from build123d import *

# Parameters (mm, degrees)
F0_R     = 25.4
F0_R_2   = 3.81
F1_DEPTH = 6.35
F2_R     = 19.05
F2_R_2   = 13.97
F3_DEPTH = 2.54
F4_R     = 2.53999


# Not quite as in the source:
# - a fillet or chamfer is up to 0.001 mm smaller than in the source, because OpenCascade refuses the exact size


with BuildPart() as f1:
    # F0 (on Front) → F1 (new body)
    with BuildSketch(Plane.XZ):
        Circle(F0_R)
        Circle(F0_R_2, mode=Mode.SUBTRACT)
    extrude(amount=F1_DEPTH)

    # F2 (on face) → F3 (cut)
    with BuildSketch(Plane.XZ.offset(6.35)):
        Circle(F2_R)
        Circle(F2_R_2, mode=Mode.SUBTRACT)
    extrude(amount=-F3_DEPTH, mode=Mode.SUBTRACT)

    # F4 (radius 2.54 in the source; OpenCascade refuses exactly that, so slightly less here)
    f4_edges = [f1.edges().sort_by_distance(p)[0] for p in [
        (-19.05, -3.81, 0),
        (-13.97, -3.81, 0),
    ]]
    fillet(f4_edges, radius=F4_R)


solid = f1.part
Geometry: final body of the model. Coordinates: model frame, mm. Coordinates: 2 decimals unless noted, no trailing zeros. Order: outer loops, then holes, each group sorted by start corner. A loop starts at its lowest first (then second) coordinate and runs counter-clockwise, first axis right, second up.
(1) Material intervals for probe 1 along X at (y, z) = (-5.5, 10); probe 2 along X at (y, z) = (-5.5, 3); probe 3 along Z at (x, y) = (5, -4.75), sorted ascending.
(2) Section query D-D (y = -1.75). Return the cut outline in (x, z).
(3) Section query C-C (y = -5). Return the cut outline in (x, z), plus the area to 3 significant figures.
(4) First-contact query: pin 1 (1.5 mm diameter, centred on y = -4.5, z = -12, fed in from +X); pin 2 (2 mm diameter, centred on y = -2.5, z = -5.5, fed in from -X); pin 3 (1 mm diameter, centred on x = -10.5, z = -2.5, fed in from +Y). Flat tips, straight axial feed; report the tip coordinate or a pass-through.
(5) Draft query along X for faces 1 (the face through (5, 0, 0)), 2 (the face through (-5.506, -3.131, -24.796)), 3 (the face through (-0.83, -3.13, -3.72)). Return one class per face: pulls with the +X half, pulls with the -X half, needs draft (parallel to the pull), parting line crosses it, or undercut.
Solution:
1. probe 1: x = -23.35 to -16.04, -9.96 to 9.96, 16.04 to 23.35
1. probe 2: x = -25.22 to -18.66, -13.79 to -2.35, 2.35 to 13.79, 18.66 to 25.22
1. probe 3: z = -24.9 to -17.79, -13.65 to 13.65, 17.79 to 24.9
2. outline: circle Ø50.8 at (0, 0); hole circle Ø7.62 at (0, 0)
3. outline: circle Ø50.8 at (0, 0); circle Ø28.72 at (0, 0); hole circle Ø37.32 at (0, 0); hole circle Ø7.62 at (0, 0)
3. area: 1,530 mm2
4. pin 1: stops at x = 22.77
4. pin 2: stops at x = -25
4. pin 3: stops at y = 0
5. face 1: needs draft
5. face 2: parting line crosses it
5. face 3: undercut
